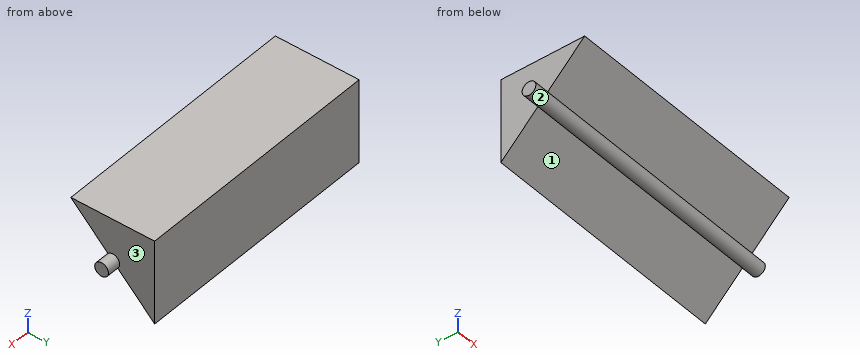
from build123d import *

# Parameters (mm, degrees)
SKETCH1_W                = 914.4
SKETCH1_H                = 304.8
BOSS_EXTRUDE1_DEPTH      = 304.8
CUT_EXTRUDE1_DEPTH       = 914.4
BOSS_EXTRUDE2_DEPTH      = 50
BOSS_EXTRUDE2_DEPTH_BACK = 976
SKETCH3_R                = 25


with BuildPart() as part:
    # Sketch1 → Boss-Extrude1 (new body)
    with BuildSketch(Plane.XY):
        Rectangle(SKETCH1_W, SKETCH1_H)
    extrude(amount=BOSS_EXTRUDE1_DEPTH)

    # Sketch2 → Cut-Extrude1 (cut)
    with BuildSketch(Plane(origin=(457.2, 0, 0), x_dir=(0, 0, -1), z_dir=(1, 0, 0))):
        Polygon((-304.8, -152.4), (0, 152.4), (0, -152.4), align=None)
    extrude(amount=-CUT_EXTRUDE1_DEPTH, mode=Mode.SUBTRACT)

    # Sketch3 → Boss-Extrude2 (add, two sides: drawn at the far end of the back side and taken through both)
    with BuildSketch(Plane(origin=(457.2, 0, 0), x_dir=(0, 0, -1), z_dir=(1, 0, 0)).offset(-BOSS_EXTRUDE2_DEPTH_BACK)):
        with Locations((-152.4, 0)):
            Circle(SKETCH3_R)
    extrude(amount=BOSS_EXTRUDE2_DEPTH + BOSS_EXTRUDE2_DEPTH_BACK)


solid = part.part
Design review of the part built by this model. Coordinates are the model's own, in mm. Face numbers are marked on the shaded views. Coordinates: 2 decimals unless noted, no trailing zeros. Write each loop counter-clockwise with the first axis right and the second up, starting at its lowest first coordinate (ties: lowest second). Pieces come first, ordered by that corner, then holes. Notation, with made-up numbers: (48.5, -17.75) - (100.5, -17.75) arc R12 ccw to (100.5, -0.75) - close; hole circle Ø9 at (-10.75, 1). An arc over 180 degrees is marked (long way). One line per item, written item: value.
1) Add section A-A (y = 0). State the section outline as (x, z) points.
Answer sheet:
outline: (-518.8, 127.4) - (507.2, 127.4) - (507.2, 177.4) - (457.2, 177.4) - (457.2, 304.8) - (-457.2, 304.8) - (-457.2, 177.4) - (-518.8, 177.4) - close
2) Insertion check: pin 1 (4 mm diameter, centred on x = -29, y = -72.5, fed in from -Z); pin 2 (1.5 mm diameter, centred on x = -210, z = 55.5, fed in from -Y); pin 3 (3 mm diameter, centred on x = -222, z = 61.5, fed in from -Y). Each pin has a flat end and moves straight along its axis. Give the tip position at first contact, or say it passes through.
Answer sheet:
pin 1: stops at z = 222.9
pin 2: stops at y = 96.15
pin 3: stops at y = 89.4
3) Add section C-C (x = -407.5). State the section outline as (y, z) points.
Answer sheet:
outline: (-152.4, 304.8) - (-17.68, 170.08) arc R25 ccw to (17.68, 134.72) - (152.4, 0) - (152.4, 304.8) - close
4) Add section D-D (z = 225). State the section outline as (x, y) points.
Answer sheet:
outline: (-457.2, -72.6) - (457.2, -72.6) - (457.2, 152.4) - (-457.2, 152.4) - close
5) To check wall thickness, follow probe 1 along X at (y, z) = (87, 290); probe 2 along Z at (x, y) = (-90, -130.5); probe 3 along Z at (x, y) = (-369, -135). State the ranges of each line that lie inside material, in increasing order.
Answer sheet:
probe 1: x = -457.2 to 457.2
probe 2: z = 282.9 to 304.8
probe 3: z = 287.4 to 304.8
6) Add section B-B (z = 152.4). State the section outline as (x, y) points.
Answer sheet:
outline: (-518.8, -25) - (507.2, -25) - (507.2, 25) - (457.2, 25) - (457.2, 152.4) - (-457.2, 152.4) - (-457.2, 25) - (-518.8, 25) - close
7) Mouldability with a two-part tool opening along Z and no side actions: class the marked faces 1, 2 and 3 as +Z half, -Z half, draft (parallel to the pull), parting line (faces both ways), or undercut.
Answer sheet:
face 1: -Z half
face 2: undercut
face 3: draft
